Work out the finished part from the listing and answer in its coordinate system (mm). A direction names the side the tool comes from. Give positions to 0.01 mm unless a question says otherwise; leave off trailing zeros. Order: outer loops, then holes, each group sorted by start corner. A loop starts at its lowest first (then second) coordinate and runs counter-clockwise, first axis right, second up. Notation, with made-up numbers: (15, -36) -> (33, -36) arc R35 cw to (33, -4) -> close; hole circle Ø8 at (-4, 49.25). An arc over 180 degrees is marked (long way). Answer as CSV lines item,"result". Start each with the question number.
1. A cutting plane is placed at D-D (x = -41). Give the vertices of the cut face in (y, z), then the cut area to 3 significant figures.
2. Flat-ended cylindrical pins translate along their axes: pin 1 (4 mm diameter, centred on x = -12, y = -50, fed in from -Z); pin 2 (10 mm diameter, centred on y = -52.5, z = 24.5, fed in from -X); pin 3 (2 mm diameter, centred on x = -10.5, y = -60, fed in from -Z). Find the tip coordinate at first contact, or state that the pin passes through.
3. Find the intervals of material crossed by L1, parallel to Y at x = 52, z = 27.5; L2, parallel to Y at x = -28, z = 2.5; L3, parallel to Z at x = 4, y = -79, in increasing order.
4. A cutting plane is placed at B-B (x = 0). Give the vertices of the cut face in (y, z).
5. A cutting plane is placed at C-C (y = -76). Give the vertices of the cut face in (x, z), then the cut area to 3 significant figures.
6. For faces 1 (the flat face through (-1, -12, -38.92)), 2 (the cylindrical face through (17.024, -35.89, 26.702)), determine the directions among +Z, -Z, +X, -X, +Y, -Y from which every point of the face is accessible in a straight line to the end or side of a thin tool.
7. A cutting plane is placed at A-A (z = 0). Give the vertices of the cut face in (x, y).
from build123d import *

# Parameters (mm, degrees)
F0_W     = 140.272602
F0_H     = 77.840932
F1_DEPTH = 23.368
F2_R     = 31.667864
F3_DEPTH = 25.4
F4_R     = 27.452249
F5_DEPTH = 25.4
F6_R     = 22.492116
F7_DEPTH = 22.86


with BuildPart() as f1:
    # F0 (on Front) → F1 (new body)
    with BuildSketch(Plane.XZ):
        Rectangle(F0_W, F0_H)
    extrude(amount=F1_DEPTH)

    # F2 (on face) → F3 (join)
    with BuildSketch(Plane.XZ.offset(23.368)):
        Circle(F2_R)
    extrude(amount=F3_DEPTH)

    # F4 (on face) → F5 (join)
    with BuildSketch(Plane.XZ.offset(48.768)):
        Circle(F4_R)
    extrude(amount=F5_DEPTH)

    # F6 (on face) → F7 (join)
    with BuildSketch(Plane.XZ.offset(74.168)):
        Circle(F6_R)
    extrude(amount=F7_DEPTH)


solid = f1.part
Answer sheet:
1,outline,"(-23.37, -38.92) -> (0, -38.92) -> (0, 38.92) -> (-23.37, 38.92) -> close"
1,area,"1,820 mm^2"
2,pin 1,"stops at z = -29.9"
2,pin 2,"stops at x = -23.55"
2,pin 3,"stops at z = -25.76"
3,L1,"y = -23.37 to 0"
3,L2,"y = -48.77 to 0"
3,L3,"z = -22.13 to 22.13"
4,outline,"(-97.03, -22.49) -> (-74.17, -22.49) -> (-74.17, -27.45) -> (-48.77, -27.45) -> (-48.77, -31.67) -> (-23.37, -31.67) -> (-23.37, -38.92) -> (0, -38.92) -> (0, 38.92) -> (-23.37, 38.92) -> (-23.37, 31.67) -> (-48.77, 31.67) -> (-48.77, 27.45) -> (-74.17, 27.45) -> (-74.17, 22.49) -> (-97.03, 22.49) -> close"
5,outline,"circle Ø44.98 at (0, 0)"
5,area,"1,590 mm^2"
6,face 1,"-Z, +X, -X, +Y, -Y"
6,face 2,"-Y"
7,outline,"(-70.14, -23.37) -> (-31.67, -23.37) -> (-31.67, -48.77) -> (-27.45, -48.77) -> (-27.45, -74.17) -> (-22.49, -74.17) -> (-22.49, -97.03) -> (22.49, -97.03) -> (22.49, -74.17) -> (27.45, -74.17) -> (27.45, -48.77) -> (31.67, -48.77) -> (31.67, -23.37) -> (70.14, -23.37) -> (70.14, 0) -> (-70.14, 0) -> close"
